from build123d import *

# Parameters (mm, degrees)
SKETCH1_R           = 7
BOSS_EXTRUDE1_DEPTH = 5


with BuildPart() as part:
    # Sketch1 → Boss-Extrude1 (new body)
    with BuildSketch(Plane.XY):
        with BuildLine():
            Line((1651.475381164, 459.392203427), (263.475381164, 459.392203427))
            Line((263.475381164, 459.392203427), (263.475381164, 834.392203427))
            ThreePointArc((263.475381164, 834.392203427), (957.475381164, 709.790289397), (1651.475381164, 834.392203427))
            Line((1651.475381164, 834.392203427), (1651.475381164, 459.392203427))
        make_face()
        with Locations((507.475381164, 484.392203427)):
            Circle(SKETCH1_R, mode=Mode.SUBTRACT)
        with Locations((807.475381164, 484.392203427)):
            Circle(SKETCH1_R, mode=Mode.SUBTRACT)
        with Locations((1107.475381164, 484.392203427)):
            Circle(SKETCH1_R, mode=Mode.SUBTRACT)
        with Locations((1407.475381164, 484.392203427)):
            Circle(SKETCH1_R, mode=Mode.SUBTRACT)
        with BuildLine():
            Line((1434.054921304, 734.606048794), (1424.329475699, 732.278881466))
            ThreePointArc((1424.329475699, 732.278881466), (1415.892646645, 737.457676261), (1421.07144144, 745.894505314))
            Line((1421.07144144, 745.894505314), (1430.796887045, 748.221672642))
            ThreePointArc((1430.796887045, 748.221672642), (1439.233716099, 743.042877847), (1434.054921304, 734.606048794))
        make_face(mode=Mode.SUBTRACT)
        with BuildLine():
            Line((1119.982718617, 684.308820718), (1110.01296021, 683.531699563))
            ThreePointArc((1110.01296021, 683.531699563), (1102.490144515, 689.966545639), (1108.924990592, 697.489361333))
            Line((1108.924990592, 697.489361333), (1118.894748999, 698.266482489))
            ThreePointArc((1118.894748999, 698.266482489), (1126.417564694, 691.831636413), (1119.982718617, 684.308820718))
        make_face(mode=Mode.SUBTRACT)
        with BuildLine():
            Line((801.909045951, 683.762551995), (791.940463281, 684.554612313))
            ThreePointArc((791.940463281, 684.554612313), (785.516897635, 692.087062405), (793.049347727, 698.510628051))
            Line((793.049347727, 698.510628051), (803.017930397, 697.718567733))
            ThreePointArc((803.017930397, 697.718567733), (809.441496043, 690.186117641), (801.909045951, 683.762551995))
        make_face(mode=Mode.SUBTRACT)
        with BuildLine():
            Line((487.665932753, 732.980693573), (477.94398541, 735.322432212))
            ThreePointArc((477.94398541, 735.322432212), (472.777839317, 743.767012399), (481.222419504, 748.933158492))
            Line((481.222419504, 748.933158492), (490.944366848, 746.591419854))
            ThreePointArc((490.944366848, 746.591419854), (496.110512941, 738.146839666), (487.665932753, 732.980693573))
        make_face(mode=Mode.SUBTRACT)
    extrude(amount=BOSS_EXTRUDE1_DEPTH)


solid = part.part
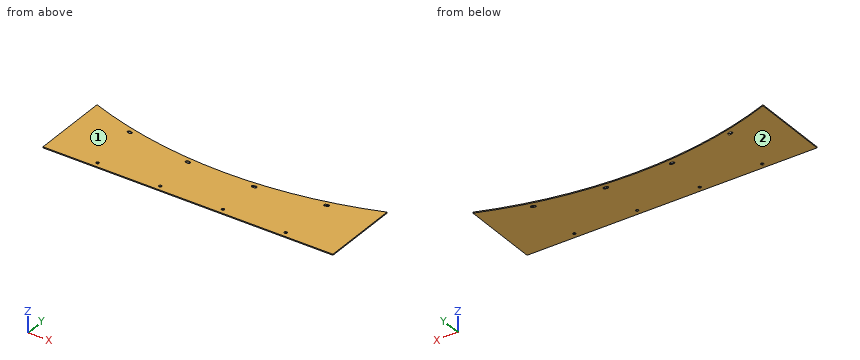
The listing builds one solid part. Answer for the finished solid, in the listing's coordinates (mm). Face numbers are marked on the shaded views. Coordinates: 2 decimals unless noted, no trailing zeros. Write each loop counter-clockwise with the first axis right and the second up, starting at its lowest first coordinate (ties: lowest second). Pieces come first, ordered by that corner, then holes. Notation, with made-up numbers: M 65,49.5 L 121,49.5 A31 cw 121,84.5 Z; hole C 31.5,11.25 d8. An arc over 180 degrees is marked long. Write each question's results on one line, items separated by ' | '.
Item 1: The part is cut by section B-B on x = 367. Determine the outline of the cut face in (y, z), and give its area (3 significant figures).
Answer below:
outline: M 459.39,0 L 799.18,0 L 799.18,5 L 459.39,5 Z | area: 1,700 mm2
Item 2: For a pull along Z with two mould halves and no side action, classify the marked faces 1 and 2 as released by +Z, released by -Z, zero draft, split by the parting line, or undercut.
Answer below:
face 1: released by +Z | face 2: released by -Z
Item 3: Consider probe 1 along Y at (x, z) = (804.5, 0.5); probe 2 along X at (y, z) = (487.5, 3.55); probe 3 along Y at (x, z) = (1431, 1.95). Determine where each line is inside the solid, lowest interval first. Write a range as [from, to].
Answer below:
probe 1: [459.39, 478.06], [490.73, 684.04], [697.44, 715.66] | probe 2: [263.48, 501.2], [513.75, 801.2], [813.75, 1101.2], [1113.75, 1401.2], [1413.75, 1651.48] | probe 3: [459.39, 733.88], [748.27, 766.8]
Item 4: The part is cut by section A-A on z = 3.4. State how many separate pieces and enclosed holes the cut face has, and give its area (3 significant figures).
Answer below:
separate pieces: 1 | enclosed holes: 8 | area: 403,000 mm2
Item 5: The part is cut by section C-C on x = 1564. Determine the outline of the cut face in (y, z).
Answer below:
outline: M 459.39,0 L 804.22,0 L 804.22,5 L 459.39,5 Z
Item 6: Given P1, Ø16, axis at x = 807.48, y = 484.39, coming from the -Z side, flat-ended and moving along its own axis, determine where the tip first touches the part or whether it passes through.
Answer below:
P1: z = 0
